For this review, take the finished solid that the model builds, in its own axes (mm). Face numbers are marked on the shaded views. A direction names the side the tool comes from. Give positions to 0.01 mm unless a question says otherwise; leave off trailing zeros. Order: outer loops, then holes, each group sorted by start corner. A loop starts at its lowest first (then second) coordinate and runs counter-clockwise, first axis right, second up. Notation, with made-up numbers: M 4,15.25 L 19,15.25 A14 cw 19,24.25 Z; hole C 4.25,15.25 d2. An arc over 180 degrees is marked long. Answer as CSV lines item,"result". Start each with the question number.
1. We need section D-D, the plane y = 18. Give the boundary of the cut face in (x, z), and give its area (3 significant figures).
2. For line 1 along X through (y, z) = (25.5, -22); line 2 along X through (y, z) = (4, 21); line 3 along Z through (x, y) = (82, -1), list the stretches that pass through material, from the lowest coordinate up.
3. We need section C-C, the plane x = 38. Give the boundary of the cut face in (y, z).
4. We need section A-A, the plane y = 0. Give the boundary of the cut face in (x, z).
5. Machinability: for the marked faces 1, 2 and 3, which of the approach directions +Z, -Z, +X, -X, +Y, -Y give a long, thin tool a straight path to every point of the face, cutting with its end or side? Answer none if there is none.
6. We need section B-B, the plane z = 0. Give the boundary of the cut face in (x, y).
7. Clearance check with flat-ended pins moving along their axes: P1, Ø2, axis at y = 31, z = 28.5, coming from the -X side; P2, Ø5.5, axis at x = 67, y = 23, coming from the -Z side; P3, Ø4, axis at y = 14, z = -26.5, coming from the +X side; P4, Ø1.5, axis at x = 32.5, z = 24.5, coming from the +Y side. State where each tip first meets the part, or that it passes through.
from build123d import *

# Parameters (mm, degrees)
CUT_EXTRUDE1_DEPTH = 40


with BuildPart() as part:
    # Sketch1 → Revolve2 (revolve)
    with BuildSketch(Plane.XY, mode=Mode.PRIVATE) as revolve2_sk:
        Polygon((30, 30), (30, 40), (40, 40), (40, 25), (80, 25), (80, 20), (110, 20), (110, 0), (51.715920118, 0), (0, 0), (0, 30), align=None)
    revolve(revolve2_sk.sketch.rotate(Axis((-14.684767441, 0, 0), (1, 0, 0)), 90), axis=Axis((-14.684767441, 0, 0), (1, 0, 0)))

    # Sketch2 → Cut-Extrude1 (cut)
    with BuildSketch(Plane(origin=(80, 0, 0), x_dir=(0, 0, -1), z_dir=(1, 0, 0))):
        with BuildLine():
            Line((-3, 24.819347292), (-3, 19.773719933))
            ThreePointArc((-3, 19.773719933), (0, 20), (3, 19.773719933))
            Line((3, 19.773719933), (3, 24.819347292))
            ThreePointArc((3, 24.819347292), (0, 25), (-3, 24.819347292))
        make_face()
    extrude(amount=-CUT_EXTRUDE1_DEPTH, mode=Mode.SUBTRACT)


solid = part.part
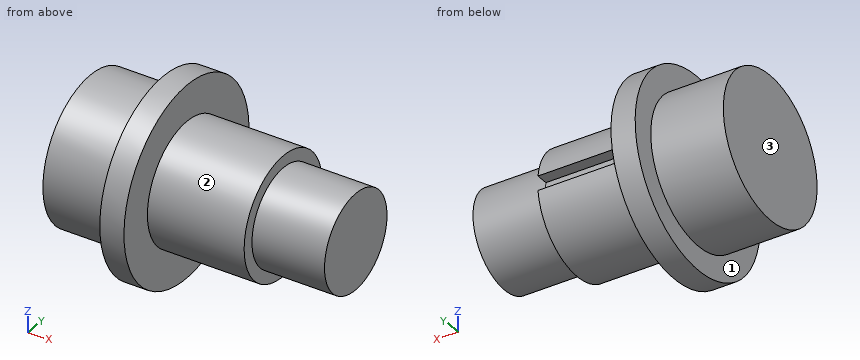
Result set:
1,outline,"M 0,-24 L 30,-24 L 30,-35.72 L 40,-35.72 L 40,-17.35 L 80,-17.35 L 80,-8.72 L 110,-8.72 L 110,8.72 L 80,8.72 L 80,17.35 L 40,17.35 L 40,35.72 L 30,35.72 L 30,24 L 0,24 Z"
1,area,"4,070 mm2"
2,line 1,"30 to 40"
2,line 2,"0 to 80"
2,line 3,"-19.97 to 19.97"
3,outline,"C 0,0 d80"
4,outline,"M 0,-30 L 30,-30 L 30,-40 L 40,-40 L 40,-25 L 80,-25 L 80,-20 L 110,-20 L 110,20 L 80,20 L 80,25 L 40,25 L 40,40 L 30,40 L 30,30 L 0,30 Z"
5,face 1,"-X"
5,face 2,"+X"
5,face 3,"+Z, -Z, -X, +Y, -Y"
6,outline,"M 0,-30 L 30,-30 L 30,-40 L 40,-40 L 40,-25 L 80,-25 L 80,-20 L 110,-20 L 110,20 L 40,20 L 40,40 L 30,40 L 30,30 L 0,30 Z"
7,P1,"through"
7,P2,"z = -14.66"
7,P3,"x = 40"
7,P4,"y = 32.19"
